```python
from build123d import *

# Parameters (mm, degrees)
F0_R     = 20
F0_W     = 22
F0_H     = 22
F0_R_2   = 10
F0_R_3   = 1.5
F0_W_2   = 8
F0_H_2   = 8
F1_DEPTH = 2
F2_D     = 3
F2_DEPTH = 25
F2_TIP   = 0.9012909285


with BuildPart() as f1:
    # F0 (on Top) → F1 (new body)
    with BuildSketch(Plane.XY):
        Circle(F0_R)
        Rectangle(F0_W, F0_H, mode=Mode.SUBTRACT)
        Rectangle(F0_W, F0_H)
        Circle(F0_R_2, mode=Mode.SUBTRACT)
        Circle(F0_R_2)
        with Locations((-7.5, 0)):
            Circle(F0_R_3, mode=Mode.SUBTRACT)
        Rectangle(F0_W_2, F0_H_2, mode=Mode.SUBTRACT)
        with Locations((7.5, 0)):
            Circle(F0_R_3, mode=Mode.SUBTRACT)
    extrude(amount=F1_DEPTH)

    # F2
    with Locations(Plane(origin=(0, 0, 0), x_dir=(1, 0, 0), z_dir=(0, 0, -1))):
        with Locations((-16.35, 0), (16.35, 0)):
            Hole(F2_D / 2, depth=F2_DEPTH)
            with Locations((0, 0, -(F2_DEPTH + F2_TIP / 2))):  # 118° drill point
                Cone(0, F2_D / 2, F2_TIP, mode=Mode.SUBTRACT)


solid = f1.part
```
Build history of the part. All positions in model axes, mm. A direction names the side the tool comes from. Give positions to 0.01 mm unless a question says otherwise; leave off trailing zeros. Loops run counter-clockwise (first coordinate to the right, second up) from the corner with the lowest first, then second, coordinate; pieces in that order, holes last.
Item 1: Pull direction Y, two halves, no side cores. Call faces 3 (the face through (0, 4, 1)), 4 (the face through (-0.3, -4.2, 2)), 5 (the face through (-9, 0, 1)), 6 (the face through (-4.336, -19.524, 0.986)): released by +Y, released by -Y, zero draft, split by the parting line, or undercut.
Answers follow:
face 3: undercut
face 4: zero draft
face 5: undercut
face 6: split by the parting line
Item 2: Which spindle directions (+Z, -Z, +X, -X, +Y, -Y) get a long thin tool onto all of the face, cutting with end or side? Do faces 1 (the face through (-0.3, -4.2, 0)), 2 (the face through (4, 0, 1)). Say none if no direction does.
Answers follow:
face 1: -Z, +X, -X, +Y, -Y
face 2: +Z, -Z
Item 3: Slice it at B-B, the plane y = 0. List the corners of the cut face in (x, z), and give its area (3 significant figures).
Answers follow:
outline: (-20, 0) - (-17.85, 0) - (-17.85, 2) - (-20, 2) - close; (-14.85, 0) - (-9, 0) - (-9, 2) - (-14.85, 2) - close; (-6, 0) - (-4, 0) - (-4, 2) - (-6, 2) - close; (4, 0) - (6, 0) - (6, 2) - (4, 2) - close; (9, 0) - (14.85, 0) - (14.85, 2) - (9, 2) - close; (17.85, 0) - (20, 0) - (20, 2) - (17.85, 2) - close
area: 40.0 mm2
Item 4: Slice it at D-D, the plane x = 16.35. List the corners of the cut face in (y, z).
Answers follow:
outline: (-11.52, 0) - (-1.5, 0) - (-1.5, 2) - (-11.52, 2) - close; (1.5, 0) - (11.52, 0) - (11.52, 2) - (1.5, 2) - close
Item 5: Drill centre lines: line 1 (Y direction, x = -16.5, z = 1.05); line 2 (Y direction, x = -1, z = 0.5); line 3 (X direction, y = -0.5, z = 0.5). Where is each one in solid material? Low to high.
Answers follow:
line 1: y = -11.3 to -1.49, 1.49 to 11.3
line 2: y = -19.97 to -4, 4 to 19.97
line 3: x = -19.99 to -17.76, -14.94 to -8.91, -6.09 to -4, 4 to 6.09, 8.91 to 14.94, 17.76 to 19.99
Item 6: Flat gauge pins, fed straight in: pin 1 (1 mm diameter, centred on x = 1.5, z = 1, fed in from -Y) (3 decimals); pin 2 (1 mm diameter, centred on x = 0.5, z = 1, fed in from +Y); pin 3 (0.6 mm diameter, centred on y = 1.5, z = 1.5, fed in from +X). Where does each tip first touch, or does it go through?
Answers follow:
pin 1: stops at y = -19.975
pin 2: stops at y = 20
pin 3: stops at x = 19.96
Item 7: Slice it at C-C, the plane z = 1.6. List the corners of the cut face in (x, y).
Answers follow:
outline: circle Ø40 at (0, 0); hole circle Ø3 at (-16.35, 0); hole circle Ø3 at (-7.5, 0); hole (-4, -4) - (4, -4) - (4, 4) - (-4, 4) - close; hole circle Ø3 at (7.5, 0); hole circle Ø3 at (16.35, 0)
Item 8: Slice it at A-A, the plane x = 0. List the corners of the cut face in (y, z), and give its area (3 significant figures).
Answers follow:
outline: (-20, 0) - (-4, 0) - (-4, 2) - (-20, 2) - close; (4, 0) - (20, 0) - (20, 2) - (4, 2) - close
area: 64.0 mm2
